The model under review builds one solid part; all positions refer to its coordinate system, in mm. Face numbers are marked on the shaded views. A direction names the side the tool comes from. Coordinates: 2 decimals unless noted, no trailing zeros. Order: outer loops, then holes, each group sorted by start corner. A loop starts at its lowest first (then second) coordinate and runs counter-clockwise, first axis right, second up.
```python
from build123d import *

# Parameters (mm, degrees)
ESQUISSE1_R                  = 2.45
BOSS_EXTRU_1_DEPTH           = 2.5
BOSS_EXTRU_4_START           = -2.5
ESQUISSE4_R                  = 10
ESQUISSE4_R_2                = 2.45
BOSS_EXTRU_4_DEPTH           = 2.5
ESQUISSE5_R                  = 0.9
ENL_V_MAT_EXTRU_3_DEPTH      = 10
R_VOLUTION1_ANGLE            = 90
R_VOLUTION1_OTHER_WAY_ANGLE  = 90
R_VOLUTION2_ANGLE            = 90
R_VOLUTION3_ANGLE            = 90
ESQUISSE9_W                  = 52
ESQUISSE9_H                  = 7.295463698
ENL_V_MAT_EXTRU_4_DEPTH      = 4
ENL_V_MAT_EXTRU_5_DEPTH      = 62.032778079
ENL_V_MAT_EXTRU_5_DEPTH_BACK = 62.032778079
ESQUISSE10_W                 = 5
ESQUISSE10_H                 = 14.990995253


with BuildPart() as part:
    # Esquisse1 → Boss.-Extru.1 (new body)
    with BuildSketch(Plane.XY):
        with BuildLine():
            Line((0, 5.147731849), (50, 5.147731849))
            ThreePointArc((50, 5.147731849), (55.147731849, 0), (50, -5.147731849))
            Line((50, -5.147731849), (0, -5.147731849))
            ThreePointArc((0, -5.147731849), (-5.147731849, 0), (0, 5.147731849))
        make_face()
        Circle(ESQUISSE1_R, mode=Mode.SUBTRACT)
        with Locations((50, 0)):
            Circle(ESQUISSE1_R, mode=Mode.SUBTRACT)
    extrude(amount=BOSS_EXTRU_1_DEPTH)

    # Esquisse4 → Boss.-Extru.4 (add)
    # profile 1 of 2: a face of its own
    with BuildSketch(Plane.XY.offset(2.5).offset(BOSS_EXTRU_4_START)):
        Circle(ESQUISSE4_R)
        Circle(ESQUISSE4_R_2, mode=Mode.SUBTRACT)
    # profile 2 of 2: a face of its own
    with BuildSketch(Plane.XY.offset(2.5).offset(BOSS_EXTRU_4_START)):
        with Locations((50, 0)):
            Circle(ESQUISSE4_R)
        with Locations((50, 0)):
            Circle(ESQUISSE4_R_2, mode=Mode.SUBTRACT)
    extrude(amount=BOSS_EXTRU_4_DEPTH)

    # Esquisse5 → Enlèv. mat.-Extru.3 (cut)
    with BuildSketch(Plane.XY.offset(2.5)):
        with Locations((-8, 0)):
            Circle(ESQUISSE5_R)
        with Locations((-5.656854249, 5.656854249)):
            Circle(ESQUISSE5_R)
        with Locations((0, 8)):
            Circle(ESQUISSE5_R)
        with Locations((0, -8)):
            Circle(ESQUISSE5_R)
        with Locations((-5.656854249, -5.656854249)):
            Circle(ESQUISSE5_R)
        with Locations((50, -8)):
            Circle(ESQUISSE5_R)
        with Locations((55.656854249, -5.656854249)):
            Circle(ESQUISSE5_R)
        with Locations((58, 0)):
            Circle(ESQUISSE5_R)
        with Locations((55.656854249, 5.656854249)):
            Circle(ESQUISSE5_R)
        with Locations((50, 8)):
            Circle(ESQUISSE5_R)
    extrude(amount=-ENL_V_MAT_EXTRU_3_DEPTH, mode=Mode.SUBTRACT)

    # Esquisse6 → Révolution1 (revolve)
    with BuildSketch(Plane(origin=(0, 0, 0), x_dir=(1, 0, 0), z_dir=(0, 1, 0))):
        Polygon((8.57326407, -6.3), (41.42673593, -6.3), (50, -6.3), (50, -7.5), (41.42673593, -7.5), (8.57326407, -7.5), (0, -7.5), (0, -6.3), align=None)
    revolve(axis=Axis((8.57326407, 0, 2.5), (1, 0, 0)), revolution_arc=R_VOLUTION1_ANGLE)

    # Esquisse6 → Révolution1 other way (revolve)
    with BuildSketch(Plane(origin=(0, 0, 0), x_dir=(1, 0, 0), z_dir=(0, 1, 0))):
        Polygon((8.57326407, -6.3), (41.42673593, -6.3), (50, -6.3), (50, -7.5), (41.42673593, -7.5), (8.57326407, -7.5), (0, -7.5), (0, -6.3), align=None)
    revolve(axis=Axis((8.57326407, 0, 2.5), (-1, 0, 0)), revolution_arc=R_VOLUTION1_OTHER_WAY_ANGLE)

    # Esquisse7 → Révolution2 (revolve)
    with BuildSketch(Plane.ZY):
        with BuildLine():
            Line((2.5, 5), (2.5, 3.8))
            ThreePointArc((2.5, 3.8), (6.3, 0), (2.5, -3.8))
            Line((2.5, -3.8), (2.5, -5))
            ThreePointArc((2.5, -5), (7.5, 0), (2.5, 5))
        make_face()
    revolve(axis=Axis((0, 5, 2.5), (0, -1, 0)), revolution_arc=R_VOLUTION2_ANGLE)

    # Esquisse8 → Révolution3 (revolve)
    with BuildSketch(Plane(origin=(50, 0, 0), x_dir=(0, 0, -1), z_dir=(1, 0, 0))):
        with BuildLine():
            Line((-2.5, 5), (-2.5, 3.8))
            ThreePointArc((-2.5, 3.8), (-6.3, 0), (-2.5, -3.8))
            Line((-2.5, -3.8), (-2.5, -5))
            ThreePointArc((-2.5, -5), (-7.5, 0), (-2.5, 5))
        make_face()
    revolve(axis=Axis((50, 5, 2.5), (0, 1, 0)), revolution_arc=R_VOLUTION3_ANGLE)

    # Esquisse9 → Enlèv. mat.-Extru.4 (cut)
    with BuildSketch(Plane(origin=(0, 0, 0), x_dir=(-1, 0, 0), z_dir=(0, 0, -1))):
        with Locations((-25, 0)):
            Rectangle(ESQUISSE9_W, ESQUISSE9_H)
    extrude(amount=-ENL_V_MAT_EXTRU_4_DEPTH, mode=Mode.SUBTRACT)

    # Esquisse10 → Enlèv. mat.-Extru.5 (cut, two sides: drawn at the far end of the back side and taken through both)
    with BuildSketch(Plane.XY.offset(2.5).offset(-ENL_V_MAT_EXTRU_5_DEPTH_BACK)):
        with Locations((0, 4.954797126)):
            Rectangle(ESQUISSE10_W, ESQUISSE10_H)
        with Locations((50, 4.954797126)):
            Rectangle(ESQUISSE10_W, ESQUISSE10_H)
    extrude(amount=ENL_V_MAT_EXTRU_5_DEPTH + ENL_V_MAT_EXTRU_5_DEPTH_BACK, mode=Mode.SUBTRACT)


solid = part.part
```
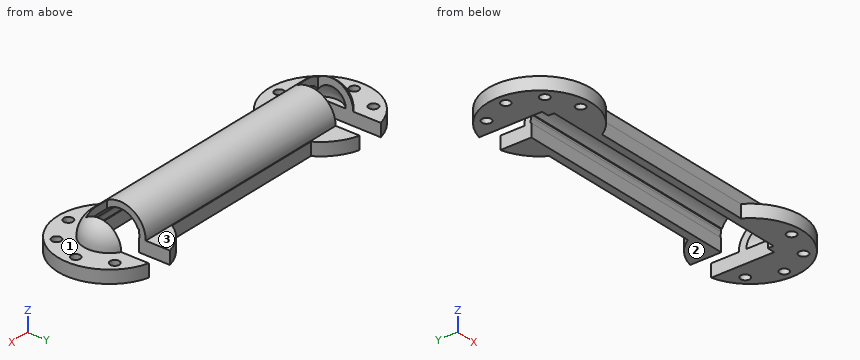
(1) We need section A-A, the plane y = -8. Write out the cut boundary in (x, z).
A:
outline: (-6, 0) - (-0.9, 0) - (-0.9, 2.5) - (-6, 2.5) - close; (0.9, 0) - (6, 0) - (6, 2.5) - (0.9, 2.5) - close; (44, 0) - (49.1, 0) - (49.1, 2.5) - (44, 2.5) - close; (50.9, 0) - (56, 0) - (56, 2.5) - (50.9, 2.5) - close
(2) For pin 1 Ø3 at (x, y) = (1.5, -1.5) entering from -Z; pin 2 Ø0.9 at (y, z) = (-3, 1) entering from +X; pin 3 Ø2 at (y, z) = (3.5, 4) entering from +X, all flat-tipped, find the tip position at first contact; note any pin that passes through.
A:
pin 1: stops at z = 4.83
pin 2: stops at x = 59.67
pin 3: stops at x = 54.14
(3) Wall thickness on probe 1 along Y at (x, z) = (28.5, 2.75); probe 2 along Y at (x, z) = (50, 0.6); probe 3 along X at (y, z) = (-0.5, 3.25): over which ranges is each line inside the solid? List them lowest first.
A:
probe 1: y = -4.99 to -3.79, 3.79 to 4.99
probe 2: y = -10 to -8.9, -7.1 to -3.65
probe 3: x = -4.92 to -3.69, 53.69 to 54.92
(4) Machinability: for the marked faces 1, 2 and 3, which of the approach directions +Z, -Z, +X, -X, +Y, -Y give a long, thin tool a straight path to every point of the face, cutting with its end or side? Answer none if there is none.
A:
face 1: +Z
face 2: -Z, +X, -X, +Y, -Y
face 3: +Z, +X, -X, +Y
(5) We need section B-B, the plane y = 0. Write out the cut boundary in (x, z), and give its area (3 significant figures).
A:
outline: (-10, 0) - (-8.9, 0) - (-8.9, 2.5) - (-10, 2.5) - close; (-7.1, 0) - (-2.5, 0) - (-2.5, 2.5) - (-3.8, 2.5) arc R3.8 cw to (-2.5, 5.36) - (-2.5, 6.83) arc R5 ccw to (-5, 2.5) - (-7.1, 2.5) - close; (2.5, 6.3) - (47.5, 6.3) - (47.5, 7.5) - (2.5, 7.5) - close; (52.5, 0) - (57.1, 0) - (57.1, 2.5) - (55, 2.5) arc R5 ccw to (52.5, 6.83) - (52.5, 5.36) arc R3.8 cw to (53.8, 2.5) - (52.5, 2.5) - close; (58.9, 0) - (60, 0) - (60, 2.5) - (58.9, 2.5) - close
area: 92.7 mm2
(6) We need section D-D, the plane x = 13.5. Write out the cut boundary in (y, z).
A:
outline: (-5.15, 0) - (-3.65, 0) - (-3.65, 2.5) - (-3.8, 2.5) arc R3.8 cw to (-3.65, 3.56) - (-3.65, 4) - (-3.49, 4) arc R3.8 cw to (3.49, 4) - (3.65, 4) - (3.65, 3.56) arc R3.8 cw to (3.8, 2.5) - (3.65, 2.5) - (3.65, 0) - (5.15, 0) - (5.15, 2.5) - (5, 2.5) arc R5 ccw to (-5, 2.5) - (-5.15, 2.5) - close
(7) We need section C-C, the plane z = 1. Count the separate pieces of the cut face and the enclosed holes in it, and give its area (3 significant figures).
A:
separate pieces: 2
enclosed holes: 8
area: 466 mm2
